```python
from build123d import *

# Parameters (mm, degrees)
EXTRUDE_2_DEPTH          = 35
EXTRUDE_3_DEPTH          = 5
CUT_EXTRUDE_1_DEPTH      = 84.440098274
CUT_EXTRUDE_1_DEPTH_BACK = 84.440098274
FILLET_1_R               = 10
SKETCH_3_W               = 5
SKETCH_3_H               = 108
EXTRUDE_4_DEPTH          = 35
CUT_EXTRUDE_2_DEPTH      = 84.440098274
CUT_EXTRUDE_2_DEPTH_BACK = 84.440098274
RIB_5_REACH              = 85.44
SKETCH_5_WALL_W          = 203.962385762
SKETCH_5_WALL_H          = 10
RIB_6_REACH              = 113.863
SKETCH_8_WALL_W          = 260.809051254
SKETCH_8_WALL_H          = 10
MIRROR_3_COPY_1_REACH    = 113.863
MIRROR_3_COPY_1_SKETCH_W = 260.809051254
MIRROR_3_COPY_1_SKETCH_H = 10
FILLET_2_R               = 2


with BuildPart() as part:
    # Sketch 1 → Extrude 2 (new body)
    with BuildSketch(Plane.XY):
        Polygon((-47.5, 42), (-47.5, -42), (-30.5, -59), (30.5, -59), (47.5, -42), (47.5, 42), (30.5, 59), (-30.5, 59), align=None)
        Polygon((-42.5, 39.5), (-42.5, -39.5), (-28, -54), (28, -54), (42.5, -39.5), (42.5, 39.5), (28, 54), (-28, 54), align=None, mode=Mode.SUBTRACT)
    extrude(amount=EXTRUDE_2_DEPTH)

    # Sketch 1_2 → Extrude 3 (add)
    # profile 1 of 2: a face of its own
    with BuildSketch(Plane.XY):
        Polygon((-47.5, 42), (-47.5, -42), (-30.5, -59), (30.5, -59), (47.5, -42), (47.5, 42), (30.5, 59), (-30.5, 59), align=None)
        Polygon((-28, 54), (-42.5, 39.5), (-42.5, -39.5), (-28, -54), (28, -54), (42.5, -39.5), (42.5, 39.5), (28, 54), align=None, mode=Mode.SUBTRACT)
    # profile 2 of 2: a face of its own
    with BuildSketch(Plane.XY):
        Polygon((28, 54), (-28, 54), (-42.5, 39.5), (-42.5, -39.5), (-28, -54), (28, -54), (42.5, -39.5), (42.5, 39.5), align=None)
    extrude(amount=-EXTRUDE_3_DEPTH)

    # Sketch 2 → Cut-Extrude 1 (cut, two sides: drawn at the far end of the back side and taken through both)
    with BuildSketch(Plane(origin=(0, 0, 0), x_dir=(0, 0, -1), z_dir=(1, 0, 0)).offset(-CUT_EXTRUDE_1_DEPTH_BACK)):
        Polygon((-27.5, -24.5), (-7.5, -24.5), (-2.5, -24.5), (-2.5, 24.5), (-7.5, 24.5), (-27.5, 24.5), align=None)
    extrude(amount=CUT_EXTRUDE_1_DEPTH + CUT_EXTRUDE_1_DEPTH_BACK, mode=Mode.SUBTRACT)

    # Fillet 1
    fillet_1_edges = [part.edges().sort_by_distance(p)[0] for p in [
        (-30.5, 59, 15),
        (30.5, 59, 15),
        (47.5, 42, 15),
        (47.5, -42, 15),
        (30.5, -59, 15),
        (-30.5, -59, 15),
        (-47.5, -42, 15),
        (-47.5, 42, 15),
    ]]
    fillet(fillet_1_edges, radius=FILLET_1_R)

    # Sketch 3 → Extrude 4 (add)
    with BuildSketch(Plane.XY):
        with Locations((17.6, 0)):
            Rectangle(SKETCH_3_W, SKETCH_3_H)
        with Locations((-17.6, 0)):
            Rectangle(SKETCH_3_W, SKETCH_3_H)
    extrude(amount=-EXTRUDE_4_DEPTH)

    # Sketch 4 → Cut-Extrude 2 (cut, two sides: drawn at the far end of the back side and taken through both)
    with BuildSketch(Plane(origin=(0, 0, 0), x_dir=(0, 0, -1), z_dir=(1, 0, 0)).offset(-CUT_EXTRUDE_2_DEPTH_BACK)):
        with BuildLine():
            Line((20, 16), (35, 16))
            Line((35, 16), (35, 24))
            Line((35, 24), (20, 24))
            ThreePointArc((20, 24), (16, 20), (20, 16))
        make_face()
        with BuildLine():
            Line((35, -16), (35, -24))
            Line((35, -24), (20, -24))
            ThreePointArc((20, -24), (16, -20), (20, -16))
            Line((20, -16), (35, -16))
        make_face()
    extrude(amount=CUT_EXTRUDE_2_DEPTH + CUT_EXTRUDE_2_DEPTH_BACK, mode=Mode.SUBTRACT)

    # Sketch 5 wall → Rib 5 (add, up to next)
    with BuildSketch(Plane(origin=(31.3, 0, -18.5), x_dir=(-0.638500632437, 0, -0.769621298027), z_dir=(-0.769621298027, 0, 0.638500632437)), mode=Mode.PRIVATE) as rib_5_sk1:
        Rectangle(SKETCH_5_WALL_W, SKETCH_5_WALL_H)
    rib_5_tool1 = extrude(rib_5_sk1.sketch, amount=RIB_5_REACH, mode=Mode.PRIVATE) - part.part
    rib_5 = rib_5_tool1.solids().sort_by_distance((31.3, 0, -18.5))[0]
    add(rib_5)

    # Mirror 1: Rib 5 across plane
    add(rib_5.mirror(Plane(origin=(0, 0, 0), x_dir=(0, 0, 1), z_dir=(1, 0, 0))))

    # Sketch 8 wall → Rib 6 (add, up to next)
    with BuildSketch(Plane(origin=(31.3, 36.037767227, -18.5), x_dir=(-0.638500632437, 0, -0.769621298027), z_dir=(-0.769621298027, 0, 0.638500632437)), mode=Mode.PRIVATE) as rib_6_sk1:
        Rectangle(SKETCH_8_WALL_W, SKETCH_8_WALL_H)
    rib_6_tool1 = extrude(rib_6_sk1.sketch, amount=RIB_6_REACH, mode=Mode.PRIVATE) - part.part
    rib_6 = rib_6_tool1.solids().sort_by_distance((31.3, 36.037767227, -18.5))[0]
    add(rib_6)

    # Mirror 2: Rib 6 across plane
    add(rib_6.mirror(Plane(origin=(0, 0, 0), x_dir=(0, 0, 1), z_dir=(1, 0, 0))))

    # Mirror 3: Rib 6 across plane
    add(rib_6.mirror(Plane.ZX))

    # Mirror 3 copy 1 sketch → Mirror 3 copy 1 (add, up to next)
    with BuildSketch(Plane(origin=(-31.3, -36.037767227, -18.5), x_dir=(0.638500632437, 0, -0.769621298027), z_dir=(0.769621298027, 0, 0.638500632437)), mode=Mode.PRIVATE) as mirror_3_copy_1_sk1:
        Rectangle(MIRROR_3_COPY_1_SKETCH_W, MIRROR_3_COPY_1_SKETCH_H)
    mirror_3_copy_1_tool1 = extrude(mirror_3_copy_1_sk1.sketch, amount=MIRROR_3_COPY_1_REACH, mode=Mode.PRIVATE) - part.part
    add(mirror_3_copy_1_tool1.solids().sort_by_distance((-31.3, -36.037767227, -18.5))[0])

    # Fillet 2
    fillet_2_edges = [part.edges().sort_by_distance(p)[0] for p in [
        (20.1, -39, -35),
        (-20.1, 39, -35),
        (-20.1, 0, -35),
        (-20.1, -39, -35),
        (20.1, 0, -35),
        (20.1, 39, -35),
    ]]
    fillet(fillet_2_edges, radius=FILLET_2_R)


solid = part.part
```
Could you check a few things on this model? Use its own coordinates, in mm. A direction names the side the tool comes from. Give positions to 0.01 mm unless a question says otherwise; leave off trailing zeros. Order: outer loops, then holes, each group sorted by start corner. A loop starts at its lowest first (then second) coordinate and runs counter-clockwise, first axis right, second up.
Q1. Suppose I cut it at D-D, the plane z = -3.5. Write out the boundary of the cut face in (x, y), and give its area (3 significant figures).
Q2. Suppose I cut it at C-C, the plane x = 4. Write out the boundary of the cut face in (y, z).
Q3. We'd pull the mould along Y, two halves only. Please class faces 1 (the flat face through (-17, 39, -35)), 2 (the cylindrical face through (-46.76, -41.63, 15.28)), 3 (the flat face through (-45, -24.5, 15)): +Y half, -Y half, draft (parallel to the pull), parting line (faces both ways), or undercut.
Q4. I'm going to push flat-ended pins straight in: P1, Ø11, axis at x = -33.5, z = -13, coming from the +Y side; P2, Ø4, axis at x = 45.5, z = 13, coming from the -Y side; P3, Ø3, axis at x = 37, z = 15.5, coming from the +Y side. Where does each tip first touch, or does it pass through?
Q5. If I drill on line 1 along Y through (x, z) = (25.5, 28); line 2 along X through (y, z) = (2.5, 0.5); line 3 along X through (y, z) = (45, -16.5), over which ranges is the centre line in solid material (lowest first)?
Q6. For faces 4 (the flat face through (-28, 31.038, -15)), 5 (the flat face through (15.1, -1, -20)), 6 (the flat face through (-18, 54, -20)), 7 (the flat face through (-45, 24.5, 15)), 8 (the flat face through (18, -24, -28)), which set-ups out of +Z, -Z, +X, -X, +Y, -Y let a thin tool reach every point of the face, with its end or its side?
Q7. Suppose I cut it at A-A, the plane y = -20. Write out the boundary of the cut face in (x, z), and give its area (3 significant figures).
Solution:
1. outline: (-47.5, -37.86) arc R10 ccw to (-44.57, -44.93) - (-33.43, -56.07) arc R10 ccw to (-26.36, -59) - (26.36, -59) arc R10 ccw to (33.43, -56.07) - (44.57, -44.93) arc R10 ccw to (47.5, -37.86) - (47.5, 37.86) arc R10 ccw to (44.57, 44.93) - (33.43, 56.07) arc R10 ccw to (26.36, 59) - (-26.36, 59) arc R10 ccw to (-33.43, 56.07) - (-44.57, 44.93) arc R10 ccw to (-47.5, 37.86) - close
1. area: 10,600 mm2
2. outline: (-59, -5) - (59, -5) - (59, 35) - (54, 35) - (54, 0) - (-54, 0) - (-54, 35) - (-59, 35) - close
3. face 1: draft
3. face 2: -Y half
3. face 3: undercut
4. P1: stops at y = 41.04
4. P2: stops at y = -46
4. P3: stops at y = 54
5. line 1: y = -59 to -54, 54 to 59
5. line 2: x = -47.5 to -42.5, 42.5 to 47.5
5. line 3: x = -20.1 to -15.1, 15.1 to 20.1
6. face 4: -Z, -X
6. face 5: -Z, +Y, -Y
6. face 6: -Z, +X, -X, +Y
6. face 7: +X, -X
6. face 8: -Z, +X, -X
7. outline: (-47.5, -5) - (-20.1, -5) - (-20.1, -16) - (-15.1, -16) - (-15.1, -5) - (15.1, -5) - (15.1, -16) - (20.1, -16) - (20.1, -5) - (47.5, -5) - (47.5, 2.5) - (42.5, 2.5) - (42.5, 0) - (-42.5, 0) - (-42.5, 2.5) - (-47.5, 2.5) - close; (-47.5, 27.5) - (-42.5, 27.5) - (-42.5, 35) - (-47.5, 35) - close; (42.5, 27.5) - (47.5, 27.5) - (47.5, 35) - (42.5, 35) - close
7. area: 685 mm2
